from build123d import *

# Parameters (mm, degrees)
F0_R     = 88.9
F0_R_2   = 3.9751
F0_R_3   = 76.2381
F0_R_4   = 73.0631
F1_DEPTH = 12.7
F2_DEPTH = 9.525
F0_R_5   = 2.15265
F3_DEPTH = 8.255


with BuildPart() as f1:
    # F0 (on Top) → F1 (new body)
    with BuildSketch(Plane.XY):
        Circle(F0_R)
        with Locations((-48.521673, -66.784353)):
            Circle(F0_R_2, mode=Mode.SUBTRACT)
        with Locations((48.521673, -66.784353)):
            Circle(F0_R_2, mode=Mode.SUBTRACT)
        with Locations((-78.509715, 25.509353)):
            Circle(F0_R_2, mode=Mode.SUBTRACT)
        Circle(F0_R_3, mode=Mode.SUBTRACT)
        with Locations((78.509715, 25.509353)):
            Circle(F0_R_2, mode=Mode.SUBTRACT)
        with Locations((0, 82.55)):
            Circle(F0_R_2, mode=Mode.SUBTRACT)
        Circle(F0_R_3)
        Circle(F0_R_4, mode=Mode.SUBTRACT)
    extrude(amount=-F1_DEPTH)

    # F0 (on Top) → F2 (cut)
    with BuildSketch(Plane.XY):
        Circle(F0_R_3)
        Circle(F0_R_4, mode=Mode.SUBTRACT)
    extrude(amount=-F2_DEPTH, mode=Mode.SUBTRACT)

    # F0 (on Top) → F3 (join)
    with BuildSketch(Plane.XY):
        with Locations((-48.521673, -66.784353)):
            Circle(F0_R_2)
        with Locations((-48.521673, -66.784353)):
            Circle(F0_R_5, mode=Mode.SUBTRACT)
        with Locations((48.521673, -66.784353)):
            Circle(F0_R_2)
        with Locations((48.521673, -66.784353)):
            Circle(F0_R_5, mode=Mode.SUBTRACT)
        with Locations((78.509715, 25.509353)):
            Circle(F0_R_2)
        with Locations((78.509715, 25.509353)):
            Circle(F0_R_5, mode=Mode.SUBTRACT)
        with Locations((0, 82.55)):
            Circle(F0_R_2)
        with Locations((0, 82.55)):
            Circle(F0_R_5, mode=Mode.SUBTRACT)
        with Locations((-78.509715, 25.509353)):
            Circle(F0_R_2)
        with Locations((-78.509715, 25.509353)):
            Circle(F0_R_5, mode=Mode.SUBTRACT)
    extrude(amount=-F3_DEPTH)


solid = f1.part
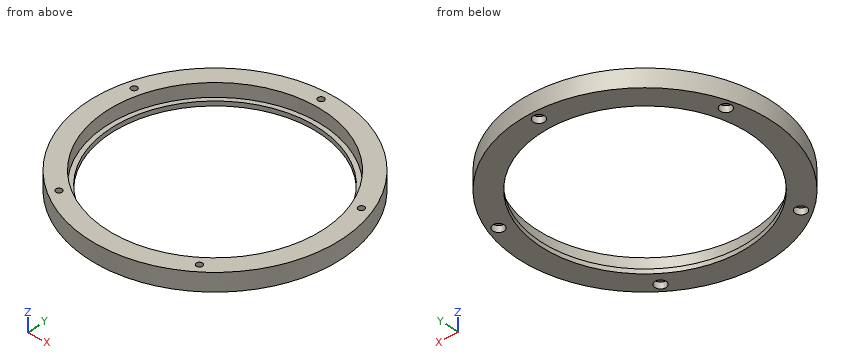
Read the model definition and answer for the solid it produces. Units are mm, in the model's axes. Coordinates: 2 decimals unless noted, no trailing zeros. Loops run counter-clockwise (first coordinate to the right, second up) from the corner with the lowest first, then second, coordinate; pieces in that order, holes last.
Q1. Consider probe 1 along Y at (x, z) = (0, -10.6); probe 2 along Y at (x, z) = (-1.5, -9.25); probe 3 along Y at (x, z) = (-22, -9). Determine where each line is inside the solid, lowest interval first.
Q2. The part is cut by section A-A on y = 0. Write down the section's boundary in (x, z) (3 decimals), and give its area (3 significant figures).
Q3. The part is cut by section B-B on x = -63. Write down the section's boundary in (y, z) (3 decimals).
Q4. The part is cut by section D-D on z = -3.25. Write down the section's boundary in (x, y).
Q5. The part is cut by section C-C on x = 0. Write down the section's boundary in (y, z) (3 decimals), and give its area (3 significant figures).
Q6. Each of these flat-tipped pins is pushed along its axis until it touches: pin 1 Ø6.5 at (x, y) = (78.51, 25.51) entering from +Z; pin 2 Ø4 at (y, z) = (-46.5, -3) entering from +X; pin 3 Ø7 at (x, y) = (78.51, 25.51) entering from -Z (3 decimals); pin 4 Ø2 at (y, z) = (12.5, -7.5) entering from +X. Where does it stop, or does it pass through?
Results below:
1. probe 1: y = -88.9 to -73.06, 73.06 to 78.57, 86.53 to 88.9
1. probe 2: y = -88.89 to -76.22, 76.22 to 78.87, 86.23 to 88.89
1. probe 3: y = -86.13 to -72.99, 72.99 to 86.13
2. outline: (-88.9, -12.7) - (-73.063, -12.7) - (-73.063, -9.525) - (-76.238, -9.525) - (-76.238, 0) - (-88.9, 0) - close; (73.063, -12.7) - (88.9, -12.7) - (88.9, 0) - (76.238, 0) - (76.238, -9.525) - (73.063, -9.525) - close
2. area: 342 mm2
3. outline: (-62.723, -12.7) - (-37.003, -12.7) - (-37.003, -9.525) - (-42.933, -9.525) - (-42.933, 0) - (-62.723, 0) - close; (37.003, -12.7) - (62.723, -12.7) - (62.723, 0) - (42.933, 0) - (42.933, -9.525) - (37.003, -9.525) - close
4. outline: circle Ø177.8 at (0, 0); hole circle Ø4.31 at (-78.51, 25.51); hole circle Ø152.48 at (0, 0); hole circle Ø4.31 at (-48.52, -66.78); hole circle Ø4.31 at (0, 82.55); hole circle Ø4.31 at (48.52, -66.78); hole circle Ø4.31 at (78.51, 25.51)
5. outline: (-88.9, -12.7) - (-73.063, -12.7) - (-73.063, -9.525) - (-76.238, -9.525) - (-76.238, 0) - (-88.9, 0) - close; (73.063, -12.7) - (78.575, -12.7) - (78.575, -8.255) - (80.397, -8.255) - (80.397, 0) - (76.238, 0) - (76.238, -9.525) - (73.063, -9.525) - close; (84.703, -8.255) - (86.525, -8.255) - (86.525, -12.7) - (88.9, -12.7) - (88.9, 0) - (84.703, 0) - close
5. area: 271 mm2
6. pin 1: stops at z = 0
6. pin 2: stops at x = 76.96
6. pin 3: stops at z = -8.255
6. pin 4: stops at x = 88.15
